Design review of the part built by this model. Coordinates are the model's own, in mm. Coordinates: 2 decimals unless noted, no trailing zeros. Write each loop counter-clockwise with the first axis right and the second up, starting at its lowest first coordinate (ties: lowest second). Pieces come first, ordered by that corner, then holes.
Q1. For pin 1 Ø6 at (x, z) = (-7, 0) entering from +Y; pin 2 Ø2 at (x, z) = (4, -1.5) entering from +Y, all flat-tipped, find the tip position at first contact; note any pin that passes through.
Q2. Take a section at B-B, the plane z = -1. Write out the cut boundary in (x, y), plus the area to 3 significant figures.
Q3. For L1, parallel to Y at x = -1.5, z = -1.75; L2, parallel to Y at x = -1, z = -0.75; L3, parallel to X at y = 46, z = 1.5, list the stretches that pass through material, from the lowest coordinate up.
Q4. The part is to be moulded in two halves that separate along X. For faces 1 (the cylindrical face through (-0.54, 47.56, -0.07)), 2 (the cylindrical face through (10, 27, 0)), 3 (the flat face through (0, 30, -5)), 4 (the cylindrical face through (0, 60, 0)), say which applies: released by +X, released by -X, zero draft, split by the parting line, or undercut.
Q5. Take a section at C-C, the plane y = 31.5. Write out the cut boundary in (x, z), plus the area to 3 significant figures.
Q6. Take a section at D-D, the plane z = 1.5. Write out the cut boundary in (x, y).
Q7. Take a section at A-A, the plane x = 0. Write out the cut boundary in (y, z), plus the area to 3 significant figures.
from build123d import *

# Parameters (mm, degrees)
SKETCH002_R  = 2.5
PAD001_DEPTH = 5
SKETCH003_R  = 10
PAD002_DEPTH = 60


with BuildPart() as lugbody:
    # Sketch002 → Pad001 (new body, symmetric)
    with BuildSketch(Plane.XY):
        with BuildLine():
            Line((-10, 0), (-10, 50))
            ThreePointArc((10, 50), (0, 60), (-10, 50))
            Line((10, 50), (10, 0))
            Line((10, 0), (-10, 0))
        make_face()
        with Locations((0, 50)):
            Circle(SKETCH002_R, mode=Mode.SUBTRACT)
    extrude(amount=PAD001_DEPTH, both=True)


with BuildPart() as lugcylinder:
    # Sketch003 → Pad002 (new body)
    with BuildSketch(Plane.XZ):
        Circle(SKETCH003_R)
    extrude(amount=-PAD002_DEPTH)

    # Boolean: intersect LugBody
    add(lugbody.part, mode=Mode.INTERSECT)


solid = lugcylinder.part
Responses:
1. pin 1: stops at y = 59.17
1. pin 2: stops at y = 59.54
2. outline: (-9.95, 0) - (9.95, 0) - (9.95, 51) arc R10 ccw to (-9.95, 51) - close; hole circle Ø5 at (0, 50)
2. area: 1,130 mm2
3. L1: y = 0 to 48, 52 to 59.89
3. L2: y = 0 to 47.71, 52.29 to 59.95
3. L3: x = -9.89 to 9.89
4. face 1: undercut
4. face 2: released by +X
4. face 3: zero draft
4. face 4: split by the parting line
5. outline: (-8.66, -5) - (8.66, -5) arc R10 ccw to (8.66, 5) - (-8.66, 5) arc R10 ccw to start
5. area: 191 mm2
6. outline: (-9.89, 0) - (9.89, 0) - (9.89, 51.5) arc R10 ccw to (-9.89, 51.5) - close; hole circle Ø5 at (0, 50)
7. outline: (0, -5) - (47.5, -5) - (47.5, 5) - (0, 5) - close; (52.5, -5) - (60, -5) - (60, 5) - (52.5, 5) - close
7. area: 550 mm2
